Check sheet for the modelled part. Datum: model origin and axes. Units: mm. Give positions to 0.01 mm unless a question says otherwise; leave off trailing zeros. Order: outer loops, then holes, each group sorted by start corner. A loop starts at its lowest first (then second) coordinate and runs counter-clockwise, first axis right, second up.
Item 1: Gauge pin test, flat ends, axial feed: P1, Ø2, axis at x = 93, y = -32, coming from the +Z side; P2, Ø1.5, axis at x = 103.5, y = -31, coming from the -Z side. Record the tip position at first contact, or that the pin passes through.
Item 2: Sectioned sample at B-B on x = 172. Record the boundary of the cut face in (y, z).
Item 3: Sectioned sample at A-A on z = 12.25. Record the boundary of the cut face in (x, y).
Item 4: Material ranges on line 1 along Y through (x, z) = (-59, 10); line 2 along Z through (x, y) = (-82.5, -28.5), recorded low to high.
from build123d import *

# Parameters (mm, degrees)
SKETCH_W          = 433
SKETCH_H          = 80
PAD_DEPTH         = 15
SKETCH001_W       = 6.5
SKETCH001_H       = 6
POCKET_DEPTH      = 216.501
POCKET_DEPTH_BACK = -216.501


with BuildPart() as part:
    # Sketch → Pad (new body)
    with BuildSketch(Plane.XY):
        Rectangle(SKETCH_W, SKETCH_H)
    extrude(amount=PAD_DEPTH)

    # Sketch001 → Pocket (cut, two sides)
    with BuildSketch(Plane.YZ) as pocket_sk:
        with Locations((-30.75, 12)):
            Rectangle(SKETCH001_W, SKETCH001_H)
    extrude(amount=-POCKET_DEPTH, mode=Mode.SUBTRACT)
    extrude(pocket_sk.sketch, amount=-POCKET_DEPTH_BACK, mode=Mode.SUBTRACT)


solid = part.part
Report:
1. P1: stops at z = 9
1. P2: stops at z = 0
2. outline: (-40, 0) - (40, 0) - (40, 15) - (-27.5, 15) - (-27.5, 9) - (-34, 9) - (-34, 15) - (-40, 15) - close
3. outline: (-216.5, -40) - (216.5, -40) - (216.5, -34) - (-216.5, -34) - close; (-216.5, -27.5) - (216.5, -27.5) - (216.5, 40) - (-216.5, 40) - close
4. line 1: y = -40 to -34, -27.5 to 40
4. line 2: z = 0 to 9
